CAD build for the part. Positions are in the model's coordinates, mm. Face numbers are marked on the shaded views. A direction names the side the tool comes from. Coordinates: 2 decimals unless noted, no trailing zeros. Order: outer loops, then holes, each group sorted by start corner. A loop starts at its lowest first (then second) coordinate and runs counter-clockwise, first axis right, second up. Notation, with made-up numbers: (-14, 36) - (9, 36) arc R21 cw to (9, 55) - close; hole circle Ø3 at (-16, 11.5). An arc over 180 degrees is marked (long way). Write each question's results on one line, items separated by ' | '. Start each with the question number.
Q1. Band-saw the part on C-C, the plane z = 4.75. Write the cut outline in (x, y), then the cut area to 3 significant figures.
Q2. Which spindle directions (+Z, -Z, +X, -X, +Y, -Y) get a long thin tool onto all of the face, cutting with end or side? Do the marked faces 5, 6, 7, 8 and 9. Say none if no direction does.
Q3. Pull direction Y, two halves, no side cores. Call the marked faces 1, 2, 3 and 4: released by +Y, released by -Y, zero draft, split by the parting line, or undercut.
Q4. Pin check, flat tips, straight feed: P1, Ø1, axis at x = 3, z = 24.5, coming from the +Y side; P2, Ø4.5, axis at y = -10, z = 45, coming from the +X side; P3, Ø12, axis at y = -10.5, z = 44.5, coming from the -X side; P4, Ø5, axis at x = 33, z = 4.5, coming from the +Y side. Stop position of each tip, or through.
Q5. Wall check: probe 1 along Y at (x, z) = (-12, 45); probe 2 along Y at (x, z) = (7.75, -24.5); probe 3 along Z at (x, y) = (6.5, 11). Give the ranges that are in metal, low to high.
Q6. Band-saw the part on D-D, the plane x = 28.5. Write the cut outline in (y, z).
Q7. Band-saw the part on A-A, the plane z = -24.5. Write the cut outline in (x, y).
Q8. Band-saw the part on B-B, the plane y = 25. Write the cut outline in (x, z), then the cut area to 3 significant figures.
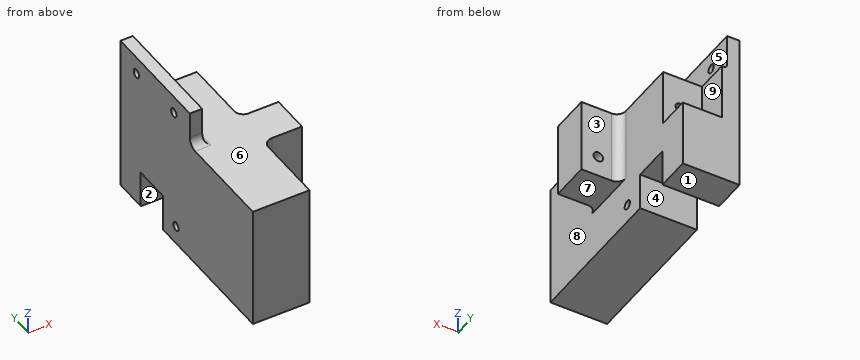
```python
from build123d import *

# Parameters (mm, degrees)
SKETCH1_W                = 32
SKETCH1_H                = 70
BOSS_EXTRUDE1_DEPTH      = 40
BOSS_EXTRUDE1_DEPTH_BACK = 84.1
SKETCH2_W                = 21
SKETCH2_H                = 21
CUT_EXTRUDE1_DEPTH       = 17
CUT_EXTRUDE1_DEPTH_BACK  = 17
CUT_EXTRUDE2_START       = -18.5
SKETCH3_W                = 22
SKETCH3_H                = 32
CUT_EXTRUDE2_DEPTH       = 18.5
SKETCH4_W                = 42
SKETCH4_H                = 22
BOSS_EXTRUDE2_DEPTH      = 22
SKETCH5_R                = 2.75
CUT_EXTRUDE3_DEPTH       = 66.6
SKETCH6_W                = 7
SKETCH6_H                = 65
BOSS_EXTRUDE3_DEPTH      = 20
SKETCH7_R                = 2.5
CUT_EXTRUDE4_DEPTH       = 17
CUT_EXTRUDE4_DEPTH_BACK  = 39
SKETCH8_R                = 2.5
CUT_EXTRUDE5_DEPTH       = 8
FILLET1_R                = 2
FILLET2_R                = 5
SKETCH9_R                = 2.5
CUT_EXTRUDE6_DEPTH       = 47.45


with BuildPart() as part:
    # Sketch1 → Boss-Extrude1 (new body, two sides)
    with BuildSketch(Plane(origin=(0, 0, 0), x_dir=(1, 0, 0), z_dir=(0, 1, 0))) as boss_extrude1_sk:
        Rectangle(SKETCH1_W, SKETCH1_H)
    extrude(amount=BOSS_EXTRUDE1_DEPTH)
    extrude(boss_extrude1_sk.sketch, amount=-BOSS_EXTRUDE1_DEPTH_BACK)

    # Sketch2 → Cut-Extrude1 (cut, two sides)
    with BuildSketch(Plane(origin=(0, 0, 0), x_dir=(0, 0, -1), z_dir=(1, 0, 0))) as cut_extrude1_sk:
        with Locations((24.5, 10.5)):
            Rectangle(SKETCH2_W, SKETCH2_H)
    extrude(amount=CUT_EXTRUDE1_DEPTH, mode=Mode.SUBTRACT)
    extrude(cut_extrude1_sk.sketch, amount=-CUT_EXTRUDE1_DEPTH_BACK, mode=Mode.SUBTRACT)

    # Sketch3 → Cut-Extrude2 (cut)
    with BuildSketch(Plane(origin=(0, 40, 0), x_dir=(1, 0, 0), z_dir=(0, 1, 0)).offset(CUT_EXTRUDE2_START)):
        with Locations((5, -19)):
            Rectangle(SKETCH3_W, SKETCH3_H)
    extrude(amount=CUT_EXTRUDE2_DEPTH, mode=Mode.SUBTRACT)

    # Sketch4 → Boss-Extrude2 (add)
    with BuildSketch(Plane(origin=(16, 0, 0), x_dir=(0, 0, -1), z_dir=(1, 0, 0))):
        with Locations((-14, -29.5)):
            Rectangle(SKETCH4_W, SKETCH4_H)
    extrude(amount=BOSS_EXTRUDE2_DEPTH)

    # Sketch5 → Cut-Extrude3 (cut, through all)
    with BuildSketch(Plane(origin=(0, -18.5, 0), x_dir=(1, 0, 0), z_dir=(0, 1, 0))):
        with Locations((28.5, -4.75)):
            Circle(SKETCH5_R)
    extrude(amount=-CUT_EXTRUDE3_DEPTH, mode=Mode.SUBTRACT)

    # Sketch6 → Boss-Extrude3 (add)
    with BuildSketch(Plane.XY.offset(35)):
        with Locations((-12.5, 7.5)):
            Rectangle(SKETCH6_W, SKETCH6_H)
    extrude(amount=BOSS_EXTRUDE3_DEPTH)

    # Sketch7 → Cut-Extrude4 (cut, two sides)
    with BuildSketch(Plane.ZY) as cut_extrude4_sk:
        with Locations((-24.5, -12)):
            Circle(SKETCH7_R)
    extrude(amount=CUT_EXTRUDE4_DEPTH, mode=Mode.SUBTRACT)
    extrude(cut_extrude4_sk.sketch, amount=-CUT_EXTRUDE4_DEPTH_BACK, mode=Mode.SUBTRACT)

    # Sketch8 → Cut-Extrude5 (cut, through all)
    with BuildSketch(Plane(origin=(-9, 0, 0), x_dir=(0, 0, -1), z_dir=(1, 0, 0))):
        with Locations((-45, 25)):
            Circle(SKETCH8_R)
        with Locations((-45, -10)):
            Circle(SKETCH8_R)
    extrude(amount=-CUT_EXTRUDE5_DEPTH, mode=Mode.SUBTRACT)

    # Fillet1
    fillet1_edges = [part.edges().sort_by_distance(p)[0] for p in [
        (-9, 7.5, 35),
    ]]
    fillet(fillet1_edges, radius=FILLET1_R)

    # Fillet2
    fillet2_edges = [part.edges().sort_by_distance(p)[0] for p in [
        (-12.5, -25, 35),
        (16, -40.5, 14),
        (16, -18.5, 14),
    ]]
    fillet(fillet2_edges, radius=FILLET2_R)

    # Sketch9 → Cut-Extrude6 (cut)
    with BuildSketch(Plane(origin=(0, 21.5, 0), x_dir=(1, 0, 0), z_dir=(0, 1, 0))):
        with Locations((6.5, -16.75)):
            Circle(SKETCH9_R)
    extrude(amount=-CUT_EXTRUDE6_DEPTH, mode=Mode.SUBTRACT)


solid = part.part
```
Results below:
1) outline: (-16, -84.1) - (16, -84.1) - (16, -45.5) arc R5 cw to (21, -40.5) - (25.75, -40.5) - (25.75, -18.5) - (21, -18.5) arc R5 cw to (16, -13.5) - (16, 21.5) - (-6, 21.5) - (-6, 40) - (-16, 40) - close; (31.25, -40.5) - (38, -40.5) - (38, -18.5) - (31.25, -18.5) - close | area: 3,940 mm²
2) face 5: +Z, +X, +Y, -Y | face 6: +Z, +X, -Y | face 7: -Z, +X, +Y, -Y | face 8: -Z, +X | face 9: +Z, +X, +Y
3) face 1: zero draft | face 2: undercut | face 3: released by +Y | face 4: undercut
4) P1: stops at y = 21.5 | P2: passes through | P3: stops at x = -16 | P4: stops at y = -18.5
5) probe 1: y = -25 to -12.5, -7.5 to 22.5, 27.5 to 40 | probe 2: y = -84.1 to -14.5, -9.5 to 0, 21 to 40 | probe 3: z = -14 to 14.25, 19.25 to 35
6) outline: (-40.5, -7) - (-18.5, -7) - (-18.5, 2) - (-40.5, 2) - close; (-40.5, 7.5) - (-18.5, 7.5) - (-18.5, 35) - (-40.5, 35) - close
7) outline: (-16, -84.1) - (16, -84.1) - (16, -14.5) - (-16, -14.5) - close; (-16, -9.5) - (16, -9.5) - (16, 0) - (-16, 0) - close; (-16, 21) - (16, 21) - (16, 40) - (-16, 40) - close
8) outline: (-16, -35) - (16, -35) - (16, 3) - (-6, 3) - (-6, 35) - (-7, 35) arc R2 cw to (-9, 37) - (-9, 42.5) - (-16, 42.5) - close; (-16, 47.5) - (-9, 47.5) - (-9, 55) - (-16, 55) - close | area: 1,640 mm²
